Geometry check sheet. Reference: the model listing, model coordinates, mm. A direction names the side the tool comes from. Give positions to 0.01 mm unless a question says otherwise; leave off trailing zeros. Loops run counter-clockwise (first coordinate to the right, second up) from the corner with the lowest first, then second, coordinate; pieces in that order, holes last. Notation, with made-up numbers: (50, 84.5) -> (74, 84.5) arc R33 cw to (74, 122.5) -> close; hole circle Ø8 at (20.25, -33.75). An arc over 180 degrees is marked (long way). Write item = value, one per line. Start each with the question number.
Autodesk Inventor part; units mm, degrees
ref_plane "Work Plane2" through (-20, 0, -10) normal (0, 0, 1) x (1, 0, 0)
ref_plane "Work Plane3" through (0, 8, 0) normal (0, 1, 0) x (1, 0, 0)
ref_plane "YZ Plane" through (0, 0, 0) normal (1, 0, 0) x (0, 1, 0)
sketch "Sketch1" plane through (0, 0, 0) normal (0, 1, 0) x (-1, 0, 0)
  line L0 (0, 0) -> (20, 0)
  line L1 (20, 0) -> (20, -20)
  line L2 (20, -20) -> (0, -20)
  line L3 (0, -20) -> (0, 0)
  dimension "d0" = 20
  dimension "d1" = 20
extrude "Extrusion1" add sketch "Sketch1" along normal blind 10
sketch "Sketch4" plane through (0, 10, 0) normal (0, 1, 0) x (1, 0, 0)
  line L0 (0, 20) -> (-20, 20)
  line L1 (-20, 20) -> (-20, 0)
  line L2 (-20, 0) -> (0, 0)
  line L3 (0, 0) -> (0, 20)
  line L4 (0, 20) -> (-20, 20)
  line L5 (-20, 20) -> (0, 0)
  line L6 (-10.1768, 10.1768) -> (-7.7019, 12.6517)
  line L7 (-7.7019, 12.6517) -> (-5.227, 10.1768)
  line L8 (-5.227, 10.1768) -> (-7.7019, 7.7019)
  line L9 (-7.7019, 7.7019) -> (-10.1768, 10.1768)
  line L10 (-10.1768, 10.1768) -> (-12.6517, 7.7019)
  line L11 (-12.6517, 7.7019) -> (-15.1265, 10.1768)
  line L12 (-15.1265, 10.1768) -> (-12.6517, 12.6517)
  line L13 (-12.6517, 12.6517) -> (-10.1768, 10.1768)
  line L14 (-12.6517, 12.6517) -> (-10.1768, 15.1265)
  line L15 (-10.1768, 15.1265) -> (-7.7019, 12.6517)
  line L16 (-7.7019, 12.6517) -> (-10.1768, 10.1768)
  line L17 (-10.1768, 10.1768) -> (-12.6517, 12.6517)
  line L18 (-12.6517, 7.7019) -> (-10.1768, 10.1768)
  line L19 (-10.1768, 10.1768) -> (-7.7019, 7.7019)
  line L20 (-7.7019, 7.7019) -> (-10.1768, 5.227)
  line L21 (-10.1768, 5.227) -> (-12.6517, 7.7019)
  dimension "d10" = 3.5
  dimension "d11" = 3.5
  dimension "d12" = 3.5
  dimension "d13" = 3.5
extrude "Extrusion3" cut sketch "Sketch4" against normal blind 8 contours L14 L15 L6 L5 | L5 L10 L11 L12 | L20 L21 L10 L5 | L5 L6 L7 L8
sketch "Sketch5" plane through (0, 10, 0) normal (0, 1, 0) x (1, 0, 0)
  line L0 (-5.227, 10.1768) -> (-10.1768, 5.227)
  line L1 (-10.1768, 5.227) -> (-15.1265, 10.1768)
  line L2 (-15.1265, 10.1768) -> (-10.1768, 15.1265)
  line L3 (-10.1768, 15.1265) -> (-5.227, 10.1768)
  line L4 (0, 20) -> (-20, 20)
  line L5 (-20, 20) -> (-20, 0)
  line L6 (-20, 0) -> (0, 0)
  line L7 (0, 0) -> (0, 20)
  line L8 (-18, 18) -> (-2, 18)
  line L9 (-2, 18) -> (-2, 2)
  line L10 (-2, 2) -> (-18, 2)
  line L11 (-18, 2) -> (-18, 18)
  line L12 (-18, 2) -> (-18, 0)
  line L13 (-2, 2) -> (-2, 0)
  line L14 (-20, 0) -> (0, 0)
  line L15 (-18, 2) -> (-20, 2)
  line L16 (-20, 20) -> (-20, 0)
  line L17 (-2, 2) -> (0, 2)
  line L18 (0, 0) -> (0, 20)
  point P0 (0, 2)
  dimension "d16" = 2
extrude "Extrusion4" add sketch "Sketch5" along normal blind 27 contours L7 L17 L9 L8 L11 L15 L5 L4
ref_plane "Work Plane1" through (-10, 10, -2) normal (1, 0, 0) x (0, 0, -1)
sketch "Sketch6" plane through (-10, 10, -2) normal (1, 0, 0) x (0, 0, -1)
  line L0 (3.227, 0) -> (8.1768, 0)
  line L1 (3.227, 0) -> (3.227, -8)
  line L2 (3.227, -8) -> (8.1768, -8)
  line L3 (8.1768, 0) -> (8.1768, -8)
  line L4 (8.1768, 0) -> (13.1265, 0)
  line L5 (8.1768, 0) -> (8.1768, -8)
  line L6 (8.1768, -8) -> (13.1265, -8)
  line L7 (13.1265, 0) -> (13.1265, -8)
  line L8 (16, 0) -> (0, 0)
  line L9 (16, 0) -> (16, 27)
  line L10 (0, 27) -> (16, 27)
  line L11 (0, 0) -> (0, 27)
  line L12 (8.1768, 0) -> (8.1768, -8)
  line L13 (8.1768, -8) -> (8.1768, -7.25)
  circle A0 centre (8.1768, -7.25) radius 0.75
  point P0 (-2, -10)
  dimension "d20" = 0.75
  dimension "d21" = 1.5
extrude "Extrusion5" cut sketch "Sketch6" along normal mid plane 27 contours A0 L3 | L3 A0
ref_plane "Work Plane2" through (-20, 0, -10) normal (0, 0, 1) x (1, 0, 0)
sketch "Sketch7" plane through (-20, 0, -10) normal (0, 0, 1) x (1, 0, 0)
  line L0 (20, 0) -> (0, 0)
  line L1 (0, 0) -> (0, 37)
  line L2 (20, 37) -> (0, 37)
  line L3 (20, 0) -> (20, 37)
  arc A0 (14.773, 3.5) -> (14.773, 2) centre (14.773, 2.75) ccw
  arc A1 (14.773, 3.5) -> (14.773, 2) centre (14.773, 2.75) ccw
  line L4 (20, 3.5) -> (20, 2)
  line L5 (20, 3.5) -> (27.5, 3.5)
  line L6 (27.5, 3.5) -> (27.5, 2)
  line L7 (27.5, 2) -> (20, 2)
  line L8 (20, 2) -> (20, 3.5)
  line L9 (20, 3.5) -> (20, 4.5)
  line L10 (20, 0) -> (20, 37)
  line L11 (27.5, 3.5) -> (27.5, 3.5246)
  line L12 (26.775, 4.2742) -> (20, 4.5)
  arc A2 (27.5, 3.5246) -> (26.775, 4.2742) centre (26.75, 3.5246) ccw
  line L13 (20, 3.5) -> (20, 2)
  line L14 (20, 2.75) -> (27.5, 2.75)
  point P0 (27.5, 4.25)
  dimension "d25" = 7.5
  dimension "d26" = 1
  dimension "d27" = 0.75
  dimension "d28" = 0.75
revolve "Revolution1" add sketch "Sketch7" angle 360 about axis through (0, 2.75, -10) along (1, 0, 0) contours L3 L12 A2 L11 L5
mirror "Mirror1" about plane through (-10, 10, -2) normal (1, 0, 0) of "Revolution1"
sketch "Sketch8" plane through (-20, 10, -2) normal (0, 0, 1) x (1, 0, 0)
  line L0 (2, 0) -> (0, 0)
  line L1 (2, 0) -> (2, 27)
  line L2 (0, 27) -> (2, 27)
  line L3 (0, 0) -> (0, 27)
  line L4 (20, 0) -> (18, 0)
  line L5 (20, 0) -> (20, 27)
  line L6 (18, 27) -> (20, 27)
  line L7 (18, 0) -> (18, 27)
  line L8 (20, 27) -> (0, 27)
  line L9 (0, 27) -> (20, 27)
  line L10 (20, 27) -> (20, 25)
  line L11 (20, 25) -> (0, 25)
  line L12 (0, 25) -> (0, 27)
  point P0 (20, -10)
  point P1 (0, 25)
  dimension "d30" = 20
  dimension "d31" = 2
extrude "Extrusion6" add sketch "Sketch8" along normal blind 2 contours L11 L3 L2 L1 | L1 L8 L7 L11 | L7 L6 L5 L11
ref_plane "Work Plane3" through (0, 8, 0) normal (0, 1, 0) x (1, 0, 0)
sketch "Sketch9" plane through (0, 8, 0) normal (0, 1, 0) x (1, 0, 0)
  line L0 (-10.1768, 15.1265) -> (-5.227, 10.1768)
  line L1 (-15.1265, 10.1768) -> (-10.1768, 15.1265)
  line L2 (-10.1768, 5.227) -> (-15.1265, 10.1768)
  line L3 (-5.227, 10.1768) -> (-10.1768, 5.227)
  line L4 (-6.6412, 10.1768) -> (-10.1768, 13.7123)
  line L5 (-10.1768, 13.7123) -> (-13.7123, 10.1768)
  line L6 (-13.7123, 10.1768) -> (-10.1768, 6.6412)
  line L7 (-10.1768, 6.6412) -> (-6.6412, 10.1768)
  point P0 (0, 0)
  dimension "d35" = 1
extrude "Extrusion7" add sketch "Sketch9" against normal blind 6
extrude "Extrusion8" cut sketch "Sketch6" along normal mid plane 27 contours A0 L3 | L3 A0
sketch "Sketch10" plane through (0, 0, 0) normal (1, 0, 0) x (0, 0, -1)
  line L0 (0, 0) -> (20, 0)
  line L1 (20, 0) -> (20, 37)
  line L2 (20, 37) -> (0, 37)
  line L3 (0, 35) -> (0, 37)
  line L4 (2, 35) -> (0, 35)
  line L5 (2, 10) -> (2, 35)
  line L6 (0, 10) -> (2, 10)
  line L7 (0, 0) -> (0, 10)
  circle A0 centre (10, 2.75) radius 1.75
  line L8 (2, 35) -> (10, 35)
  line L9 (10, 35) -> (4.5, 35)
  line L10 (4.5, 35) -> (4.5, 30)
  line L11 (4.5, 30) -> (17, 30)
  line L12 (17, 30) -> (17, 17.5)
  line L13 (17, 17.5) -> (4.5, 17.5)
  line L14 (4.5, 17.5) -> (4.5, 30)
  dimension "d40" = 5.5
  dimension "d41" = 5
  dimension "d42" = 12.5
  dimension "d43" = 12.5
  dimension "d44" = 8
extrude "Extrusion9" cut sketch "Sketch10" against normal blind 6 contours L11 L12 L13 L14
move faces "Move1" translate (0, -3, 0) faces at (-8.5269, 8, -13.0052)
move faces "Move3" translate (0, -3, 0) faces at (-5.8013, 10, -5.8013)
sketch "Sketch12" plane through (-10, 10, -2) normal (1, 0, 0) x (0, 0, -1)
  circle A0 centre (8, -7.25) radius 0.75
  point P0 (-2, -10)
extrude "Extrusion10" cut sketch "Sketch12" along normal mid plane 100
sketch "Sketch13" plane through (0, 0, 0) normal (1, 0, 0) x (0, 0, -1)
  arc A0 (10.0884, 3.4948) -> (10, 2) centre (10, 2.75) ccw
  circle A1 centre (10, 2.75) radius 1.75
  point P0 (0, 0)
  dimension "d58" = 3.5
properties part number "latticeChamberv6b"
1) Section check A-A (x = -16). Enter the section's corners in (y, z).
2) Depth check by flat-ended pin: pin 1 Ø1.5 at (x, z) = (-3, -7) entering from +Y; pin 2 Ø12 at (y, z) = (16, -15) entering from +X; pin 3 Ø10 at (y, z) = (26, -2) entering from -X; pin 4 Ø2.5 at (y, z) = (2.75, -10.18) entering from -X. Enter the tip coordinate at first touch or a pass-through.
3) Thickness scan on line 1 (X direction, y = 15, z = -6.75); line 2 (Y direction, x = -2.75, z = -10); line 3 (Z direction, x = -16, y = 2.75). Record the ranges inside material, lowest first.
4) Section check D-D (y = 34). Enter the section's corners in (x, z), plus the area to 3 significant figures.
5) Tool access check on faces 4 (the flat face through (-1, 30, -11)), 5 (the flat face through (-10, 18, -20)), 6 (the flat face through (-19, 21, -2)), 7 (the flat face through (-10, 36, -2)). Record the directions out of +Z, -Z, +X, -X, +Y, -Y that give a thin tool (end or side, any length) a straight path to the whole face; none if there is none.
6) Section check C-C (x = -11). Enter the section's corners in (y, z).
7) Draft check along Y on faces 1 (the flat face through (-8.434, 3.521, -8.384)), 2 (the flat face through (-10, 35, -1)), 3 (the conical face through (3.34, 1.542, -11.107)). Enter one of: released by +Y, released by -Y, zero draft, split by the parting line, or undercut.
8) Section check B-B (y = 27.5). Enter the section's corners in (x, z).
Check result:
q1.outline = (0, -20) -> (37, -20) -> (37, -18) -> (7, -18) -> (7, 0) -> (0, 0) -> close; (35, -2) -> (37, -2) -> (37, 0) -> (35, 0) -> close; hole (2.01, -10.09) arc R0.75 ccw (long way) to (3.49, -10.09) arc R0.75 ccw (long way) to start
q2.pin_1 = 7
q2.pin_2 = 0
q2.pin_3 = -20
q2.pin_4 = -27.5
q3.line_1 = -20 to -18, -2 to 0
q3.line_2 = 0 to 2, 3.5 to 7
q3.line_3 = -20 to -10.93, -9.25 to 0
q4.outline = (-20, -20) -> (0, -20) -> (0, -2) -> (-2, -2) -> (-2, -18) -> (-18, -18) -> (-18, -2) -> (-20, -2) -> close
q4.area = 104 mm2
q5.face_4 = +X
q5.face_5 = -Z, +X, -X, +Y, -Y
q5.face_6 = +Z, +X, -X
q5.face_7 = +Y
q6.outline = (0, -20) -> (37, -20) -> (37, -18) -> (7, -18) -> (7, -14.3) -> (5, -14.3) -> (5, -12.89) -> (2, -12.89) -> (2, -7.46) -> (5, -7.46) -> (5, -6.05) -> (7, -6.05) -> (7, 0) -> (0, 0) -> close; (35, -2) -> (37, -2) -> (37, 0) -> (35, 0) -> close
q7.face_1 = zero draft
q7.face_2 = undercut
q7.face_3 = split by the parting line
q8.outline = (-20, -20) -> (0, -20) -> (0, -17) -> (-2, -17) -> (-2, -18) -> (-18, -18) -> (-18, -2) -> (-20, -2) -> close; (-2, -4.5) -> (0, -4.5) -> (0, -2) -> (-2, -2) -> close
